Study the drawing (mm; zero at the part's minimum x, y, z) and answer. Coordinates: 2 decimals unless noted, no trailing zeros. Loops run counter-clockwise (first coordinate to the right, second up) from the corner with the lowest first, then second, coordinate; pieces in that order, holes last.
Q1. Section C-C (z = 7.25) is taken. Give the vertices of the cut face in (x, y).
Q2. Section B-B (y = 20) is taken. Give the vertices of the cut face in (x, z), then the cut area to 4 significant figures.
Q3. Section D-D (y = 93.5) is taken. Give the vertices of the cut face in (x, z).
Q4. Straight lines are drawn through the part: line 1 (Y direction, x = 87.5, z = 6.25); line 2 (Y direction, x = 83.5, z = 4.5); line 3 (X direction, y = 6, z = 2.25). For each, find the intervals that lie inside material, in ascending order.
Q5. Flat-ended cylindrical pins translate along their axes: P1, Ø6, axis at x = 95.5, y = 32, coming from the -Z side; P2, Ø10, axis at x = 87.5, y = 80, coming from the +Z side. Find the tip coordinate at first contact, or state that the pin passes through.
Q6. Section A-A (x = 87.5) is taken. Give the vertices of the cut face in (y, z).
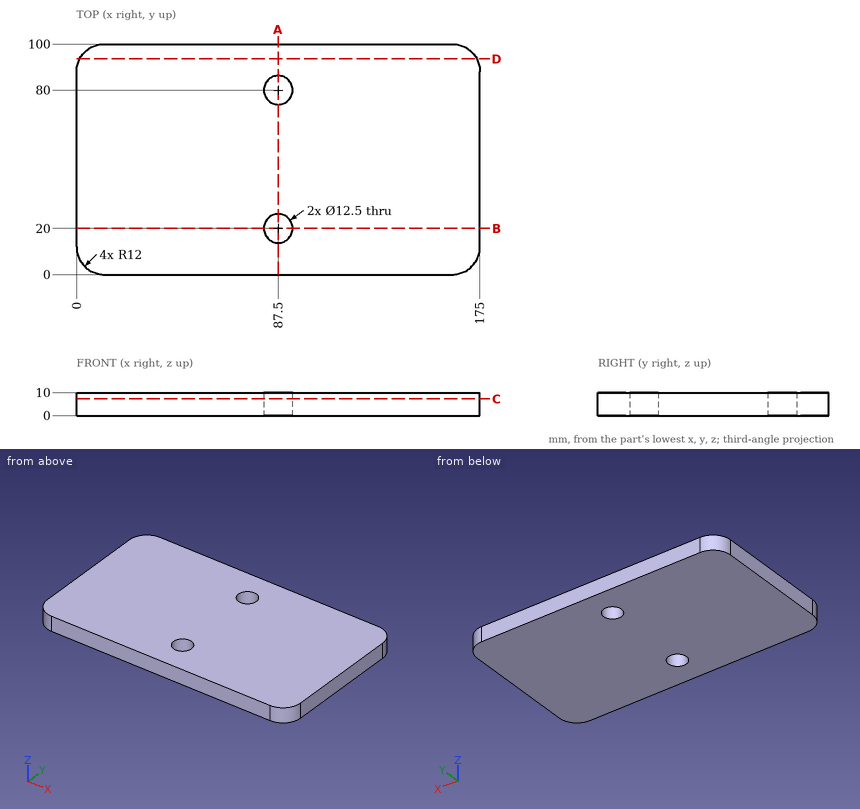
Numbers:
1. outline: (0, 12) arc R12 ccw to (12, 0) - (163, 0) arc R12 ccw to (175, 12) - (175, 88) arc R12 ccw to (163, 100) - (12, 100) arc R12 ccw to (0, 88) - close; hole circle Ø12.5 at (87.5, 20); hole circle Ø12.5 at (87.5, 80)
2. outline: (0, 0) - (81.25, 0) - (81.25, 10) - (0, 10) - close; (93.75, 0) - (175, 0) - (175, 10) - (93.75, 10) - close
2. area: 1,625 mm2
3. outline: (1.33, 0) - (173.67, 0) - (173.67, 10) - (1.33, 10) - close
4. line 1: y = 0 to 13.75, 26.25 to 73.75, 86.25 to 100
4. line 2: y = 0 to 15.2, 24.8 to 75.2, 84.8 to 100
4. line 3: x = 1.61 to 173.39
5. P1: stops at z = 0
5. P2: passes through
6. outline: (0, 0) - (13.75, 0) - (13.75, 10) - (0, 10) - close; (26.25, 0) - (73.75, 0) - (73.75, 10) - (26.25, 10) - close; (86.25, 0) - (100, 0) - (100, 10) - (86.25, 10) - close
